The model under review builds one solid part; all positions refer to its coordinate system, in mm. Face numbers are marked on the shaded views. A direction names the side the tool comes from. Give positions to 0.01 mm unless a question says otherwise; leave off trailing zeros. Order: outer loops, then holes, each group sorted by start corner. A loop starts at its lowest first (then second) coordinate and runs counter-clockwise, first axis right, second up. Notation, with made-up numbers: (-1.75, 35) - (27.25, 35) arc R15 cw to (27.25, 63) - close; hole circle Ø3 at (23, 45). An arc over 180 degrees is marked (long way). Use a Markdown table: item, result. Add a question column.
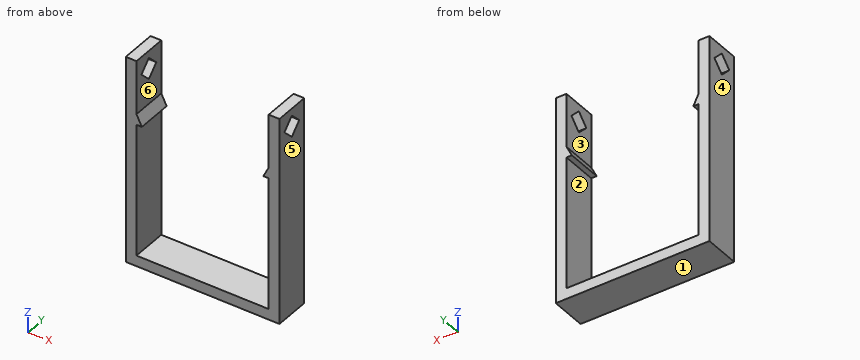
```python
from build123d import *

# Parameters (mm, degrees)
SKETCH1_W           = 3
SKETCH1_H           = 15
BOSS_EXTRUDE1_DEPTH = 10
CUT_EXTRUDE1_DEPTH  = 58.282196187


with BuildPart() as part:
    # Sketch1 → Boss-Extrude1 (new body)
    with BuildSketch(Plane(origin=(0, 0, 0), x_dir=(1, 0, 0), z_dir=(0, 1, 0))):
        Polygon((18.5, -18.5), (18.5, 18.5), (-18.5, 18.5), (-18.5, -18.5), (-18.5, -21.5), (-21.5, -21.5), (-21.5, 21.5), (21.5, 21.5), (21.5, -21.5), (18.5, -21.5), align=None)
        with Locations((-20, -29)):
            Rectangle(SKETCH1_W, SKETCH1_H)
        with Locations((20, -29)):
            Rectangle(SKETCH1_W, SKETCH1_H)
        Polygon((-18.5, -21.5), (-17, -18.5), (-18.5, -18.5), align=None)
        Polygon((17, -18.5), (18.5, -18.5), (18.5, -21.5), align=None)
    extrude(amount=BOSS_EXTRUDE1_DEPTH)

    # Sketch3 → Cut-Extrude1 (cut, through all)
    with BuildSketch(Plane(origin=(21.5, 0, 0), x_dir=(0, 0, -1), z_dir=(1, 0, 0))):
        Polygon((-31.5, 8), (-34.5, 5), (-31.5, 2), (-28.5, 5), align=None)
    extrude(amount=-CUT_EXTRUDE1_DEPTH, mode=Mode.SUBTRACT)


solid = part.part
```
Q1. We need section C-C (z = -13). Write out the cut boundary in (x, y), plus the area to 3 significant figures.
Q2. We need section B-B (z = 30). Write out the cut boundary in (x, y), plus the area to 3 significant figures.
Q3. Machinability: for the marked faces 1, 2 and 3, which of the approach directions +Z, -Z, +X, -X, +Y, -Y give a long, thin tool a straight path to every point of the face, cutting with its end or side? Answer none if there is none.
Q4. Wall thickness on probe 1 along X at (y, z) = (3.5, 26); probe 2 along Z at (x, y) = (6.5, 9); probe 3 along X at (y, z) = (9.75, 20): over which ranges is each line inside the solid? List them lowest first.
Q5. We need section D-D (y = 9). Write out the cut boundary in (x, z), plus the area to 4 significant figures.
Q6. We need section A-A (y = 4). Write out the cut boundary in (x, z), plus the area to 4 significant figures.
Q7. Clearance check with flat-ended pins moving along their axes: P1, Ø2, axis at x = 16.5, z = -3.5, coming from the +Y side; P2, Ø5, axis at x = 1.5, y = 8, coming from the +Z side; P3, Ø5, axis at y = 2.5, z = 31.5, coming from the -X side. State where each tip first meets the part, or that it passes through.
Q8. Draft analysis for pull direction X (two halves, no side actions). For the marked faces 4, 5 and 6, state which applies: pulls with the +X half, pulls with the -X half, needs draft (parallel to the pull), parting line crosses it, or undercut.
Here are the results:
| question | item | result |
|---|---|---|
| 1 | outline | (-21.5, 0) - (-18.5, 0) - (-18.5, 10) - (-21.5, 10) - close; (18.5, 0) - (21.5, 0) - (21.5, 10) - (18.5, 10) - close |
| 1 | area | 60.0 mm2 |
| 2 | outline | (-21.5, 0) - (-18.5, 0) - (-18.5, 3.5) - (-21.5, 3.5) - close; (-21.5, 6.5) - (-18.5, 6.5) - (-18.5, 10) - (-21.5, 10) - close; (18.5, 0) - (21.5, 0) - (21.5, 3.5) - (18.5, 3.5) - close; (18.5, 6.5) - (21.5, 6.5) - (21.5, 10) - (18.5, 10) - close |
| 2 | area | 42.0 mm2 |
| 3 | face 1 | -Z, +X, -X, +Y, -Y |
| 3 | face 2 | +Y, -Y |
| 3 | face 3 | +Z, +Y, -Y |
| 4 | probe 1 | -21.5 to -18.5, 18.5 to 21.5 |
| 4 | probe 2 | -21.5 to -18.5 |
| 4 | probe 3 | -21.5 to -17.75, 17.75 to 21.5 |
| 5 | outline | (-21.5, -21.5) - (21.5, -21.5) - (21.5, 36.5) - (18.5, 36.5) - (18.5, 21.5) - (17, 18.5) - (18.5, 18.5) - (18.5, -18.5) - (-18.5, -18.5) - (-18.5, 18.5) - (-17, 18.5) - (-18.5, 21.5) - (-18.5, 36.5) - (-21.5, 36.5) - close |
| 5 | area | 463.5 mm2 |
| 6 | outline | (-21.5, -21.5) - (21.5, -21.5) - (21.5, 29.5) - (18.5, 29.5) - (18.5, 21.5) - (17, 18.5) - (18.5, 18.5) - (18.5, -18.5) - (-18.5, -18.5) - (-18.5, 18.5) - (-17, 18.5) - (-18.5, 21.5) - (-18.5, 29.5) - (-21.5, 29.5) - close; (-21.5, 33.5) - (-18.5, 33.5) - (-18.5, 36.5) - (-21.5, 36.5) - close; (18.5, 33.5) - (21.5, 33.5) - (21.5, 36.5) - (18.5, 36.5) - close |
| 6 | area | 439.5 mm2 |
| 7 | P1 | through |
| 7 | P2 | z = -18.5 |
| 7 | P3 | x = -21.5 |
| 8 | face 4 | pulls with the -X half |
| 8 | face 5 | pulls with the +X half |
| 8 | face 6 | undercut |
